from build123d import *

# Parameters (mm, degrees)
SKETCH_R      = 17.7
SKETCH_R_2    = 1.5
PAD_DEPTH     = 2
SKETCH001_R   = 4
SKETCH001_R_2 = 1.15
PAD001_DEPTH  = 7.7
SKETCH002_W   = 55
SKETCH002_H   = 90.8
SKETCH002_W_2 = 51
SKETCH002_H_2 = 36
SKETCH002_H_3 = 23.4
PAD002_DEPTH  = 4
SKETCH003_W   = 45.416033
SKETCH003_H   = 18.722532
SKETCH003_W_2 = 8.527091
SKETCH003_H_2 = 17.424923
POCKET_DEPTH  = 2.001


with BuildPart() as part:
    # Sketch → Pad (new body)
    with BuildSketch(Plane.XY.offset(2)):
        Polygon((-19.3, 49.399), (-10.1, 49.399), (-10.1, 45.401), (10.1, 45.401), (10.1, 49.399), (19.3, 49.399), (19.3, 45.399), (27.5, 45.399), (27.5, -45.401), (19.3, -45.401), (19.3, -49.399), (10.1, -49.399), (10.1, -45.401), (-10.1, -45.401), (-10.1, -49.399), (-19.3, -49.399), (-19.3, -45.649884), (-27.5, -45.649884), (-27.5, 45.399), (-19.3, 45.399), align=None)
        Circle(SKETCH_R, mode=Mode.SUBTRACT)
        with Locations((-21, 0)):
            Circle(SKETCH_R_2, mode=Mode.SUBTRACT)
        with Locations((21, 0)):
            Circle(SKETCH_R_2, mode=Mode.SUBTRACT)
    extrude(amount=PAD_DEPTH)

    # Sketch001 → Pad001 (new body)
    with BuildSketch(Plane.XY.offset(4)):
        with Locations((15.45, -27.6)):
            Circle(SKETCH001_R)
        with Locations((15.45, -27.6)):
            Circle(SKETCH001_R_2, mode=Mode.SUBTRACT)
        with Locations((-8.7, -31.3)):
            Circle(SKETCH001_R)
        with Locations((-8.7, -31.3)):
            Circle(SKETCH001_R_2, mode=Mode.SUBTRACT)
    extrude(amount=PAD001_DEPTH)

    # Sketch002 → Pad002 (new body)
    with BuildSketch(Plane.XY.offset(4)):
        Rectangle(SKETCH002_W, SKETCH002_H)
        Rectangle(SKETCH002_W_2, SKETCH002_H_2, mode=Mode.SUBTRACT)
        with Locations((0, 31.7)):
            Rectangle(SKETCH002_W_2, SKETCH002_H_3, mode=Mode.SUBTRACT)
        with Locations((0, -31.7)):
            Rectangle(SKETCH002_W_2, SKETCH002_H_3, mode=Mode.SUBTRACT)
    extrude(amount=PAD002_DEPTH)

    # Sketch003 → Pocket (cut, through all)
    with BuildSketch(Plane.XY.offset(4)):
        with Locations((0.020594, 31.420495)):
            Rectangle(SKETCH003_W, SKETCH003_H)
        with Locations((-18.794618, -31.513151)):
            Rectangle(SKETCH003_W_2, SKETCH003_H_2)
        Polygon((-0.998942, -22.80069), (7.898897, -22.80069), (7.898897, -34.479092), (21.987135, -34.479092), (21.987135, -40.225613), (-0.998942, -40.225613), align=None)
    extrude(amount=-POCKET_DEPTH, mode=Mode.SUBTRACT)


solid = part.part
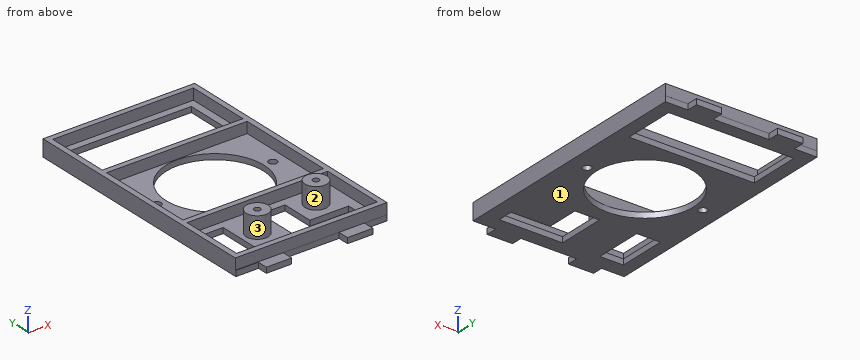
Verification items for the finished model (mm, model axes). Face numbers are marked on the shaded views. Give positions to 0.01 mm unless a question says otherwise; leave off trailing zeros. Order: outer loops, then holes, each group sorted by start corner. A loop starts at its lowest first (then second) coordinate and runs counter-clockwise, first axis right, second up. Notation, with made-up numbers: M 44.5,-20.75 L 76.5,-20.75 A23 cw 76.5,1.25 Z; hole C 29,-14 d5. An arc over 180 degrees is marked long. Answer as a JSON object with one key per item and string values. Group by question number.
1) Mould release check, pull along X, two halves, no side actions. Record for the marked faces 1, 2 and 3: released by +X, released by -X, zero draft, split by the parting line, or undercut.
2) Depth check by flat-ended pin: pin 1 Ø0.6 at (x, z) = (24, 2.5) entering from -Y; pin 2 Ø2 at (x, z) = (-19.5, 7.5) entering from +Y; pin 3 Ø1.6 at (y, z) = (-46.5, 2.5) entering from -X. Enter the tip coordinate at first touch or a pass-through.
3) Scan lines: line 1 along Y through (x, z) = (22.5, 6.5); line 2 along Y through (x, z) = (0, 3.55); line 3 along X through (y, z) = (39, 3.5). Record each from-to range of solid material in increasing order. Write a range as [from, to].
4) Cross-section at B-B (y = 0). Enter the section's corners in (x, z), then the cut area to 3 significant figures.
5) Cross-section at A-A (x = -21). Give the number of separate pieces and of enclosed holes in the cut face, then the cut area to 3 significant figures.
Result sheet:
{
 "1": {"face 1": "zero draft", "face 2": "undercut", "face 3": "undercut"},
 "2": {"pin 1": "stops at y = -45.4", "pin 2": "stops at y = 45.4", "pin 3": "stops at x = -19.3"},
 "3": {"line 1": "y = [-45.4, -43.4], [-20, -18], [18, 20], [43.4, 45.4]", "line 2": "y = [-45.4, -40.23], [-22.8, -17.7], [17.7, 22.06], [40.78, 45.4]", "line 3": "x = [-27.5, -22.69], [22.73, 27.5]"},
 "4": {"outline": "M -27.5,2 L -22.5,2 L -22.5,4 L -25.5,4 L -25.5,8 L -27.5,8 Z; M -19.5,2 L -17.7,2 L -17.7,4 L -19.5,4 Z; M 17.7,2 L 19.5,2 L 19.5,4 L 17.7,4 Z; M 22.5,2 L 27.5,2 L 27.5,8 L 25.5,8 L 25.5,4 L 22.5,4 Z", "area": "43.2 mm2"},
 "5": {"separate pieces": "4", "enclosed holes": "0", "area": "136 mm2"}
}
